Geometry check sheet. Reference: the model listing, model coordinates, mm. A direction names the side the tool comes from. Give positions to 0.01 mm unless a question says otherwise; leave off trailing zeros. Order: outer loops, then holes, each group sorted by start corner. A loop starts at its lowest first (then second) coordinate and runs counter-clockwise, first axis right, second up.
Autodesk Inventor part; units mm, degrees
ref_plane "YZ Plane" through (0, 0, 0) normal (1, 0, 0) x (0, 1, 0)
ref_plane "XZ Plane" through (0, 0, 0) normal (0, 1, 0) x (-1, 0, 0)
ref_plane "XY Plane" through (0, 0, 0) normal (0, 0, 1) x (1, 0, 0)
sketch "Sketch1" plane through (0, 0, 0) normal (0, 1, 0) x (-1, 0, 0)
  line L0 (6.35, -3.6662) -> (0, -7.3323)
  line L1 (0, -7.3323) -> (-6.35, -3.6662)
  line L2 (-6.35, -3.6662) -> (-6.35, 3.6662)
  line L3 (-6.35, 3.6662) -> (0, 7.3323)
  line L4 (0, 7.3323) -> (6.35, 3.6662)
  line L5 (6.35, 3.6662) -> (6.35, -3.6662)
  point P0 (0, 0)
  point P1 (0, 0)
  point P2 (0, 0)
  dimension "d0" = 12.7
extrude "Extrusion1" add sketch "Sketch1" along normal blind 117.475
sketch "Sketch2" plane through (0, 0, 0) normal (0, -1, 0) x (1, 0, 0)
  point P0 (0, 0)
  point P1 (0, 0)
hole "Hole1" at (0, 0, 0) direction (0, 1, 0) diameter 4.9784 depth 25.4
sketch "Sketch3" plane through (0, 117.475, 0) normal (0, 1, 0) x (1, 0, 0)
  point P0 (0, 0)
  point P1 (0, 0)
hole "Hole2" at (0, 117.475, 0) direction (0, -1, 0) diameter 4.9784 depth 25.4
properties part number "SHOT_1_009_HexShaft4" material "Aluminum 6061"
Item 1: Sectioned sample at B-B (z = 0). Enter the section's corners in (x, y) (3 decimals), and give its area (3 significant figures).
Reported:
outline: (-6.35, 0) - (-2.489, 0) - (-2.489, 25.4) - (2.489, 25.4) - (2.489, 0) - (6.35, 0) - (6.35, 117.475) - (2.489, 117.475) - (2.489, 92.075) - (-2.489, 92.075) - (-2.489, 117.475) - (-6.35, 117.475) - close
area: 1,240 mm2
Item 2: Scan lines: L1, parallel to Z at x = 0, y = 110; L2, parallel to X at y = 11, z = 0; L3, parallel to X at y = 109, z = -1. Record each from-to range of solid material in increasing order.
Reported:
L1: z = -7.33 to -2.49, 2.49 to 7.33
L2: x = -6.35 to -2.49, 2.49 to 6.35
L3: x = -6.35 to -2.28, 2.28 to 6.35
Item 3: Gauge pin test, flat ends, axial feed: pin 1 (4.5 mm diameter, centred on x = 0, z = 0, fed in from +Y) (3 decimals); pin 2 (4 mm diameter, centred on x = 0, z = 0, fed in from -Y); pin 3 (5 mm diameter, centred on x = 0.5, z = -3, fed in from -Y); pin 4 (2 mm diameter, centred on x = -3, y = 48.5, fed in from +Z). Record the tip position at first contact, or that the pin passes through.
Reported:
pin 1: stops at y = 92.075
pin 2: stops at y = 25.4
pin 3: stops at y = 0
pin 4: stops at z = 6.18
Item 4: Sectioned sample at D-D (x = 3.75). Enter the section's corners in (y, z) (3 decimals), and give its area (3 significant figures).
Reported:
outline: (0, -5.167) - (117.475, -5.167) - (117.475, 5.167) - (0, 5.167) - close
area: 1,210 mm2
Item 5: Sectioned sample at A-A (y = 14.5). Enter the section's corners in (x, z).
Reported:
outline: (-6.35, -3.67) - (0, -7.33) - (6.35, -3.67) - (6.35, 3.67) - (0, 7.33) - (-6.35, 3.67) - close; hole circle Ø4.98 at (0, 0)
Item 6: Set-up check for faces 1 (the flat face through (0, 117.475, -3)), 2 (the cylindrical face through (-0.748, 104.597, 2.374)), 3 (the flat face through (0, 25.4, 0)): record each of +Z, -Z, +X, -X, +Y, -Y from which the full face is reachable in a straight line by a thin tool's end or side.
Reported:
face 1: +Z, -Z, +X, -X, +Y
face 2: +Y
face 3: -Y
Item 7: Draft check along Z on faces 4 (the flat face through (-6.35, 58, 0)), 5 (the flat face through (3.131, 57.915, -5.525)), 6 (the flat face through (0, 92.075, 0)). Enter one of: released by +Z, released by -Z, zero draft, split by the parting line, or undercut.
Reported:
face 4: zero draft
face 5: released by -Z
face 6: undercut
Item 8: Sectioned sample at C-C (y = 38.5). Enter the section's corners in (x, z), and give its area (3 significant figures).
Reported:
outline: (-6.35, -3.67) - (0, -7.33) - (6.35, -3.67) - (6.35, 3.67) - (0, 7.33) - (-6.35, 3.67) - close
area: 140 mm2
